For this review, take the finished solid that the model builds, in its own axes (mm). A direction names the side the tool comes from. Coordinates: 2 decimals unless noted, no trailing zeros. Write each loop counter-clockwise with the first axis right and the second up, starting at its lowest first coordinate (ties: lowest second). Pieces come first, ordered by that corner, then holes.
```python
from build123d import *

# Parameters (mm, degrees)
SKETCH1_W           = 5.8
SKETCH1_H           = 5.8
BOSS_EXTRUDE1_DEPTH = 2.9


with BuildPart() as part:
    # Sketch1 → Boss-Extrude1 (new body)
    with BuildSketch(Plane.XY):
        Rectangle(SKETCH1_W, SKETCH1_H)
    extrude(amount=BOSS_EXTRUDE1_DEPTH)

    # Loft1: read off the stored shape, not the designer's step
    # Loft1: loft between two sections, ruled curve by curve
    loft1_from = [
        Edge.make_bspline([(0.877386601, 1.090959556, 16.4), (3.059305712, -0.663813647, 16.4), (1.30453251, -2.845732758, 16.4), (-0.877386601, -1.090959556, 16.4), (-3.059305712, 0.663813647, 16.4), (-1.30453251, 2.845732758, 16.4), (0.877386601, 1.090959556, 16.4)], [0, 0, 0, 0, 0.5, 0.5, 0.5, 1, 1, 1, 1], 3, [1, 0.333333333, 0.333333333, 1, 0.333333333, 0.333333333, 1]),
    ]
    loft1_to = [
        Edge.make_bspline([(1.548183001, 0.918220777, 2.9), (3.384624555, -2.178145225, 2.9), (0.288258553, -4.014586779, 2.9), (-1.548183001, -0.918220777, 2.9), (-3.384624555, 2.178145225, 2.9), (-0.288258553, 4.014586779, 2.9), (1.548183001, 0.918220777, 2.9)], [0, 0, 0, 0, 0.5, 0.5, 0.5, 1, 1, 1, 1], 3, [1, 0.333333333, 0.333333333, 1, 0.333333333, 0.333333333, 1]),
    ]
    loft1 = Solid(Shell([*[Face.make_surface_from_curves(loft1_from[k], loft1_to[k]) for k in range(1)], Face(Wire(loft1_from)), Face(Wire(loft1_to))]))
    add(loft1)


solid = part.part
```
Q1. Draft analysis for pull direction Z (two halves, no side actions). For faces 3 (the flat face through (0, 0, 0)), 4 (the flat face through (2.9, 0, 1)), 5 (the flat face through (0, 0, 16.4)), state which applies: +Z half, -Z half, draft (parallel to the pull), parting line (faces both ways), or undercut.
Ans:
face 3: -Z half
face 4: draft
face 5: +Z half
Q2. For probe 1 along Z at (x, y) = (-2.3, -2); probe 2 along X at (y, z) = (-0.1, 7.75); probe 3 along X at (y, z) = (0.75, 6.25), list the stretches that pass through material, from the lowest coordinate up.
Ans:
probe 1: z = 0 to 2.9
probe 2: x = -1.63 to 1.63
probe 3: x = -1.51 to 1.51
Q3. Tool access review of faces 1 (the flat face through (-2, 1, 2.9)), 2 (the flat face through (-2.9, 0, 1)): name each direction out of +Z, -Z, +X, -X, +Y, -Y from which nothing blocks a thin tool from reaching the whole face with its end or side.
Ans:
face 1: +Z
face 2: +Z, -Z, -X, +Y, -Y
Q4. Add section A-A (x = 2.2). State the section outline as (y, z) points, then the cut area to 3 significant figures.
Ans:
outline: (-2.9, 0) - (2.9, 0) - (2.9, 2.9) - (-2.9, 2.9) - close
area: 16.8 mm2
Q5. Clearance check with flat-ended pins moving along their axes: pin 1 Ø2 at (x, z) = (2, 6.5) entering from -Y; pin 2 Ø1.5 at (y, z) = (-1, 11.5) entering from +X; pin 3 Ø1.5 at (x, z) = (-0.5, 4.5) entering from -Y. State where each tip first meets the part, or that it passes through.
Ans:
pin 1: stops at y = -1.34
pin 2: stops at x = 1.5
pin 3: stops at y = -1.76
